Source: CAD feature listing. Evaluate the final solid. Frame: model axes, mm. A direction names the side the tool comes from. Coordinates: 2 decimals unless noted, no trailing zeros. Loops run counter-clockwise (first coordinate to the right, second up) from the corner with the lowest first, then second, coordinate; pieces in that order, holes last.
from build123d import *

# Parameters (mm, degrees)
SKETCH1_W               = 7.5
SKETCH1_H               = 7.5
SKETCH1_R               = 1.5
BOSS_EXTRUDE1_DEPTH     = 1.5
SKETCH1_3_W             = 7.5
SKETCH1_3_H             = 7.5
SKETCH1_3_R             = 1.5
BOSS_EXTRUDE2_DEPTH     = 8
SKETCH2_W               = 10
SKETCH2_H               = 25
BOSS_EXTRUDE3_DEPTH     = 35
CUT_EXTRUDE1_DEPTH      = 100.181515037
CUT_EXTRUDE1_DEPTH_BACK = 65
SKETCH4_R               = 2
CUT_EXTRUDE2_DEPTH      = 65
FILLET1_R               = 7.5


with BuildPart() as part:
    # Sketch1 → Boss-Extrude1 (new, symmetric)
    # profile 1 of 5: a face of its own
    with BuildSketch(Plane.XY):
        Polygon((-58.92, -31.87), (-58.92, -39.37), (58.92, -39.37), (58.92, -31.87), (66.42, -31.87), (66.42, 31.87), (58.92, 31.87), (58.92, 39.37), (-58.92, 39.37), (-58.92, 31.87), (-66.42, 31.87), (-66.42, -31.87), align=None)
    # profile 2 of 5: a face of its own
    with BuildSketch(Plane.XY):
        with Locations((-62.67, -35.62)):
            Rectangle(SKETCH1_W, SKETCH1_H)
        with Locations((-63.75, -36.7)):
            Circle(SKETCH1_R, mode=Mode.SUBTRACT)
    # profile 3 of 5: a face of its own
    with BuildSketch(Plane.XY):
        with Locations((-62.67, 35.62)):
            Rectangle(SKETCH1_W, SKETCH1_H)
        with Locations((-63.75, 36.7)):
            Circle(SKETCH1_R, mode=Mode.SUBTRACT)
    # profile 4 of 5: a face of its own
    with BuildSketch(Plane.XY):
        with Locations((62.67, 35.62)):
            Rectangle(SKETCH1_W, SKETCH1_H)
        with Locations((63.75, 36.7)):
            Circle(SKETCH1_R, mode=Mode.SUBTRACT)
    # profile 5 of 5: a face of its own
    with BuildSketch(Plane.XY):
        with Locations((62.67, -35.62)):
            Rectangle(SKETCH1_W, SKETCH1_H)
        with Locations((63.75, -36.7)):
            Circle(SKETCH1_R, mode=Mode.SUBTRACT)
    extrude(amount=BOSS_EXTRUDE1_DEPTH, both=True)

    # Sketch1<3> → Boss-Extrude2 (add)
    # profile 1 of 4: a face of its own
    with BuildSketch(Plane.XY):
        with Locations((-62.67, -35.62)):
            Rectangle(SKETCH1_3_W, SKETCH1_3_H)
        with Locations((-63.75, -36.7)):
            Circle(SKETCH1_3_R, mode=Mode.SUBTRACT)
    # profile 2 of 4: a face of its own
    with BuildSketch(Plane.XY):
        with Locations((-62.67, 35.62)):
            Rectangle(SKETCH1_3_W, SKETCH1_3_H)
        with Locations((-63.75, 36.7)):
            Circle(SKETCH1_3_R, mode=Mode.SUBTRACT)
    # profile 3 of 4: a face of its own
    with BuildSketch(Plane.XY):
        with Locations((62.67, 35.62)):
            Rectangle(SKETCH1_3_W, SKETCH1_3_H)
        with Locations((63.75, 36.7)):
            Circle(SKETCH1_3_R, mode=Mode.SUBTRACT)
    # profile 4 of 4: a face of its own
    with BuildSketch(Plane.XY):
        with Locations((62.67, -35.62)):
            Rectangle(SKETCH1_3_W, SKETCH1_3_H)
        with Locations((63.75, -36.7)):
            Circle(SKETCH1_3_R, mode=Mode.SUBTRACT)
    extrude(amount=BOSS_EXTRUDE2_DEPTH)

    # Sketch2 → Boss-Extrude3 (add)
    with BuildSketch(Plane(origin=(0, 0, -1.5), x_dir=(-1, 0, 0), z_dir=(0, 0, -1))):
        with Locations((-11.975, -26.87)):
            Rectangle(SKETCH2_W, SKETCH2_H)
        with Locations((11.975, -26.87)):
            Rectangle(SKETCH2_W, SKETCH2_H)
    extrude(amount=BOSS_EXTRUDE3_DEPTH)

    # Sketch3 → Cut-Extrude1 (cut, two sides: drawn at the far end of the back side and taken through both)
    with BuildSketch(Plane.ZY.offset(16.975).offset(-CUT_EXTRUDE1_DEPTH_BACK)):
        Polygon((-36.5, -14.37), (-36.5, -39.37), (-1.5, -14.37), align=None)
    extrude(amount=CUT_EXTRUDE1_DEPTH + CUT_EXTRUDE1_DEPTH_BACK, mode=Mode.SUBTRACT)

    # Sketch4 → Cut-Extrude2 (cut)
    with BuildSketch(Plane(origin=(16.975, 0, 0), x_dir=(0, 0, -1), z_dir=(1, 0, 0))):
        with Locations((16.5, -31.37)):
            Circle(SKETCH4_R)
    extrude(amount=-CUT_EXTRUDE2_DEPTH, mode=Mode.SUBTRACT)

    # Fillet1
    fillet1_edges = [part.edges().sort_by_distance(p)[0] for p in [
        (11.975, -39.37, -36.5),
        (-11.975, -39.37, -36.5),
    ]]
    fillet(fillet1_edges, radius=FILLET1_R)


solid = part.part
Q1. Access query for faces 1 (the flat face through (-58.92, 36, 5)), 2 (the flat face through (-1, 1, -1.5)), 3 (the flat face through (-63, 31.87, 5)). Directions: +Z, -Z, +X, -X, +Y, -Y. A direction counts if a zero-diameter tool reaches every point of the face in a straight line with its end or side. Return the directions, or none.
Q2. Draft query along Z for faces 4 (the cylindrical face through (12.045, -33.322, -16.066)), 5 (the flat face through (-63, -35, 8)), 6 (the flat face through (58.92, 36, 5)). Return one class per face: +Z half, -Z half, draft (parallel to the pull), parting line (faces both ways), or undercut.
Q3. Section C-C, the plane y = -36.7. Return the cut outline in (x, z) (3 decimals), plus the area to 3 significant figures.
Q4. Section B-B, the plane z = -16. Return the cut outline in (x, y) (1 decimal).
Q5. Section A-A, the plane x = 63.75. Return the cut outline in (y, z).
Q6. Section D-D, the plane x = -53. Return the cut outline in (y, z).
Q7. Contact query for flat-ended pins moving along their axis: pin 1 Ø2 at (x, y) = (-22, -12.5) entering from -Z; pin 2 Ø5 at (x, y) = (-11, -29.5) entering from -Z; pin 3 Ø6.5 at (y, z) = (-31.37, -16.5) entering from -X (3 decimals); pin 4 Ø9.5 at (y, z) = (-20.5, -9) entering from +X (3 decimals). Output: stop coordinate, or through.
Q8. Line query: line 1 along Y through (x, z) = (63.75, 0.5); line 2 along X through (y, z) = (-21.5, -8.5) (3 decimals); line 3 along Z through (x, y) = (-58, 2.5). Output: solid intervals per line, ascending.
Derived:
1. face 1: +Z, +Y, -Y
1. face 2: -Z, +Y
1. face 3: +Z, +X, -X
2. face 4: undercut
2. face 5: +Z half
2. face 6: draft
3. outline: (-66.42, -1.5) - (-65.25, -1.5) - (-65.25, 8) - (-66.42, 8) - close; (-62.25, -1.5) - (-16.975, -1.5) - (-16.975, -18.834) - (-6.975, -18.834) - (-6.975, -1.5) - (6.975, -1.5) - (6.975, -18.834) - (16.975, -18.834) - (16.975, -1.5) - (62.25, -1.5) - (62.25, 8) - (58.92, 8) - (58.92, 1.5) - (-58.92, 1.5) - (-58.92, 8) - (-62.25, 8) - close; (65.25, -1.5) - (66.42, -1.5) - (66.42, 8) - (65.25, 8) - close
3. area: 786 mm2
4. outline: (-17, -38.8) - (-7, -38.8) - (-7, -33.3) - (-17, -33.3) - close; (-17, -29.4) - (-7, -29.4) - (-7, -24.7) - (-17, -24.7) - close; (7, -38.8) - (17, -38.8) - (17, -33.3) - (7, -33.3) - close; (7, -29.4) - (17, -29.4) - (17, -24.7) - (7, -24.7) - close
5. outline: (-39.37, -1.5) - (-38.2, -1.5) - (-38.2, 8) - (-39.37, 8) - close; (-35.2, -1.5) - (35.2, -1.5) - (35.2, 8) - (31.87, 8) - (31.87, 1.5) - (-31.87, 1.5) - (-31.87, 8) - (-35.2, 8) - close; (38.2, -1.5) - (39.37, -1.5) - (39.37, 8) - (38.2, 8) - close
6. outline: (-39.37, -1.5) - (39.37, -1.5) - (39.37, 1.5) - (-39.37, 1.5) - close
7. pin 1: stops at z = -1.5
7. pin 2: stops at z = -20.6
7. pin 3: stops at x = -16.975
7. pin 4: stops at x = 16.975
8. line 1: y = -39.37 to -38.2, -35.2 to 35.2, 38.2 to 39.37
8. line 2: x = -16.975 to -6.975, 6.975 to 16.975
8. line 3: z = -1.5 to 1.5
